Here's how the part is built. I have some questions about the finished solid (model axes, mm). Coordinates: 2 decimals unless noted, no trailing zeros. Write each loop counter-clockwise with the first axis right and the second up, starting at its lowest first coordinate (ties: lowest second). Pieces come first, ordered by that corner, then holes. Notation, with made-up numbers: (-30.75, 61) -> (19.25, 61) arc R22 ccw to (19.25, 72) -> close; hole circle Ø11 at (-26.75, -16). An arc over 180 degrees is marked (long way). Put each result on its own line as item: value. Start each with the question number.
Item 1: I need wall thicknesses on line 1 (X direction, y = 16, z = 820); line 2 (Z direction, x = 1149.5, y = 14); line 3 (Z direction, x = 699.5, y = 12.5). Which ranges of each line are inside material? Lowest first, please. Write a range as [from, to].
Item 2: I want a section at B-B, the plane x = 1107.5. List the corners of the cut face in (y, z) for me.
Item 3: I want a section at C-C, the plane z = 428.5. List the corners of the cut face in (x, y) for me.
Item 4: For pin 1 (5 mm diameter, centred on x = 1177.5, y = -4, fed in from -Z); pin 2 (1.5 mm diameter, centred on y = -7.5, z = 253.5, fed in from -X); pin 3 (6 mm diameter, centred on y = 10, z = 330.5, fed in from +X); pin 4 (10 mm diameter, centred on x = 258, y = -10, fed in from -Z), each with a flat end and sliding along its axis, tell me the tip position at first contact or that it passes through.
from build123d import *

# Parameters (mm, degrees)
F1_DEPTH = 19.05


with BuildPart() as f1:
    # F0 (on Front) → F1 (new body, symmetric)
    with BuildSketch(Plane.XZ):
        Polygon((266.7, 944.5625), (0, 944.5625), (0, 792.1625), (1090.318143, 0), (1333.5, 0), (1333.5, 188.9125), (1066.8, 188.9125), (1066.8, 377.825), (800.1, 377.825), (800.1, 566.7375), (533.4, 566.7375), (533.4, 755.65), (266.7, 755.65), align=None)
    extrude(amount=F1_DEPTH, both=True)


solid = f1.part
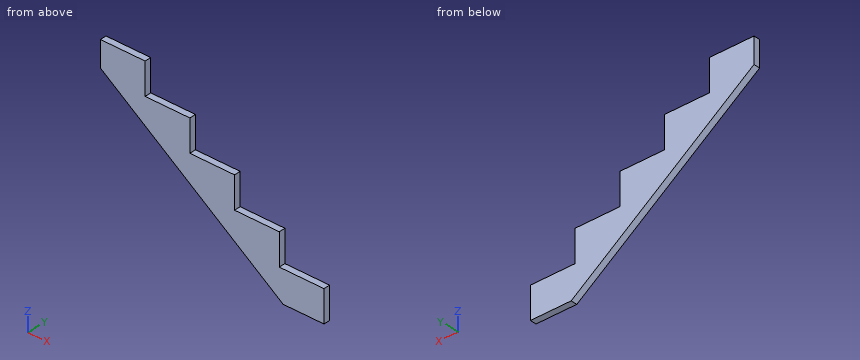
Calculated:
1. line 1: x = [0, 266.7]
1. line 2: z = [0, 188.91]
1. line 3: z = [283.95, 566.74]
2. outline: (-19.05, 0) -> (19.05, 0) -> (19.05, 188.91) -> (-19.05, 188.91) -> close
3. outline: (500.54, -19.05) -> (800.1, -19.05) -> (800.1, 19.05) -> (500.54, 19.05) -> close
4. pin 1: stops at z = 0
4. pin 2: stops at x = 740.37
4. pin 3: stops at x = 1066.8
4. pin 4: stops at z = 601.08
